from build123d import *

# Parameters (mm, degrees)
SKETCH1_W                                        = 211.932606224
SKETCH1_H                                        = 131.01903931
BOSS_EXTRUDE1_DEPTH                              = 25.4
CBORE_FOR_3_8_SOCKET_HEAD_CAP_SCREW1_D           = 10.0838
CBORE_FOR_3_8_SOCKET_HEAD_CAP_SCREW1_CBORE_D     = 15.875
CBORE_FOR_3_8_SOCKET_HEAD_CAP_SCREW1_CBORE_DEPTH = 9.525


with BuildPart() as part:
    # Sketch1 → Boss-Extrude1 (new body)
    with BuildSketch(Plane(origin=(0, 0, 0), x_dir=(1, 0, 0), z_dir=(0, 1, 0))):
        Rectangle(SKETCH1_W, SKETCH1_H)
    extrude(amount=BOSS_EXTRUDE1_DEPTH)

    # CBORE for 3/8 Socket Head Cap Screw1 (through all)
    with Locations(Plane(origin=(0, 25.4, 0), x_dir=(1, 0, 0), z_dir=(0, 1, 0))):
        with Locations((-80.566303112, -40.109519655), (-80.566303112, 40.109519655), (80.566303112, 40.109519655), (80.566303112, -40.109519655), (0, 0)):
            CounterBoreHole(CBORE_FOR_3_8_SOCKET_HEAD_CAP_SCREW1_D / 2, CBORE_FOR_3_8_SOCKET_HEAD_CAP_SCREW1_CBORE_D / 2, CBORE_FOR_3_8_SOCKET_HEAD_CAP_SCREW1_CBORE_DEPTH)


solid = part.part
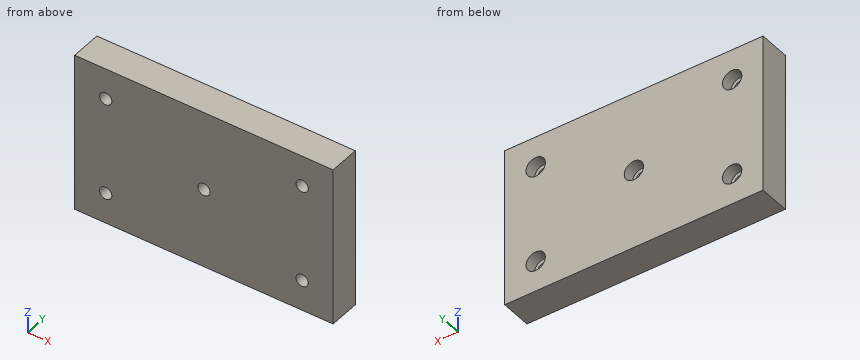
Design review of the part built by this model. Coordinates are the model's own, in mm. Round coordinates to 2 decimals unless told otherwise and drop trailing zeros. Loops run counter-clockwise (first coordinate to the right, second up) from the corner with the lowest first, then second, coordinate; pieces in that order, holes last. Notation, with made-up numbers: (69.5, 64.5) - (123.5, 64.5) arc R19 cw to (123.5, 78.5) - close; hole circle Ø11 at (51.25, -23.5). An arc over 180 degrees is marked (long way). One line per item, written item: value. Start each with the question number.
1) Consider section B-B on x = 0. Give the boundary of the cut face in (y, z) (1 decimal), then the cut area to 3 significant figures.
2) Consider section C-C on y = 22.25. Give the boundary of the cut face in (x, z) (1 decimal), then the cut area to 3 significant figures.
3) Consider section A-A on z = 0. Give the boundary of the cut face in (x, y) (1 decimal).
4) Insertion check: pin 1 Ø9.5 at (x, z) = (0, 0) entering from -Y; pin 2 Ø12.5 at (x, z) = (-79.5, 40) entering from +Y (3 decimals). Each pin has a flat end and moves straight along its axis. Give the tip position at first contact, or say it passes through.
5) To check wall thickness, follow L1, parallel to Z at x = -82.5, y = 4.75; L2, parallel to X at y = 9.5, z = -38.5; L3, parallel to Z at x = -75.5, y = 20.25. State the ranges of each line that lie inside material, in increasing order. Write a range as from..to.
Reported:
1. outline: (0, -65.5) - (25.4, -65.5) - (25.4, -7.9) - (15.9, -7.9) - (15.9, -5) - (0, -5) - close; (0, 5) - (15.9, 5) - (15.9, 7.9) - (25.4, 7.9) - (25.4, 65.5) - (0, 65.5) - close
1. area: 3,020 mm^2
2. outline: (-106, -65.5) - (106, -65.5) - (106, 65.5) - (-106, 65.5) - close; hole circle Ø15.9 at (-80.6, -40.1); hole circle Ø15.9 at (-80.6, 40.1); hole circle Ø15.9 at (0, 0); hole circle Ø15.9 at (80.6, -40.1); hole circle Ø15.9 at (80.6, 40.1)
2. area: 26,800 mm^2
3. outline: (-106, 0) - (-5, 0) - (-5, 15.9) - (-7.9, 15.9) - (-7.9, 25.4) - (-106, 25.4) - close; (5, 0) - (106, 0) - (106, 25.4) - (7.9, 25.4) - (7.9, 15.9) - (5, 15.9) - close
4. pin 1: passes through
4. pin 2: stops at y = 15.875
5. L1: z = -65.51..-44.77, -35.45..35.45, 44.77..65.51
5. L2: x = -105.97..-85.34, -75.79..75.79, 85.34..105.97
5. L3: z = -65.51..-46.22, -34..34, 46.22..65.51
